Here's how the part is built. I have some questions about the finished solid (model axes, mm). A direction names the side the tool comes from. Coordinates: 2 decimals unless noted, no trailing zeros. Write each loop counter-clockwise with the first axis right and the second up, starting at its lowest first coordinate (ties: lowest second). Pieces come first, ordered by that corner, then holes. Notation, with made-up numbers: (82.25, 39.5) -> (122.25, 39.5) arc R22 cw to (122.25, 45.5) -> close; hole circle Ø9 at (8, -1.5). An arc over 180 degrees is marked (long way). Use a Markdown table: item, result. Add a question column.
Item 1: If I drill on line 1 along X through (y, z) = (3.6, 0); line 2 along Y through (x, z) = (20.75, 1.25); line 3 along Z through (x, y) = (13.25, 13), over which ranges is the centre line in solid material (lowest first)? Write a range as from..to.
Item 2: Imagine slicing it at A-A, the plane z = 0. Write out the boundary of the cut face in (x, y), and give its area (3 significant figures).
Item 3: On a 3-axis mill with a long thin cutter (end or side, diameter ignored), from which of +Z, -Z, +X, -X, +Y, -Y can I reach the whole of each face in a straight line? I mean faces 4 (the flat face through (11, 2, 5.715)), 5 (the cylindrical face through (14.415, 12.671, 1.58)). Say none if no direction works.
Item 4: Will these pins go through, and if not, where does the flat tip stop? pin 1 Ø1.5 at (x, z) = (1, -1.5) entering from +Y; pin 2 Ø8 at (x, y) = (10, 13) entering from +Z (3 decimals); pin 3 Ø1.5 at (x, z) = (0, 0) entering from -Y; pin 4 Ø5 at (y, z) = (5.5, 4) entering from +X.
Item 5: If we mould it in two halves opening along Y, with no side actions, what happens to faces 1 (the flat face through (10, 0, 0)), 2 (the cylindrical face through (12.11, 14.61, -4.7)), 3 (the cylindrical face through (-2.11, 2.25, 0.13))? For each: pulls with the +Y half, pulls with the -Y half, needs draft (parallel to the pull), parting line crosses it, or undercut.
Item 6: Imagine slicing it at C-C, the plane x = 0. Write out the boundary of the cut face in (y, z).
Item 7: Imagine slicing it at D-D, the plane z = -1.5. Write out the boundary of the cut face in (x, y).
```python
from build123d import *

# Parameters (mm, degrees)
SKETCH1_R               = 1.2192
BOSS_EXTRUDE1_DEPTH     = 4.572
SKETCH1_3_R             = 5.625
SKETCH1_3_R_2           = 4.125
BOSS_EXTRUDE2_DEPTH     = 21
SKETCH2_R               = 1.63195
CUT_EXTRUDE1_DEPTH      = 18.923
CUT_EXTRUDE1_DEPTH_BACK = 18.923


with BuildPart() as part:
    # Sketch1 → Boss-Extrude1 (new body)
    with BuildSketch(Plane(origin=(0, 0, 0), x_dir=(1, 0, 0), z_dir=(0, 1, 0))):
        with BuildLine():
            Line((3.6045, 5.715), (17.6045, 5.715))
            ThreePointArc((17.6045, 5.715), (23.3195, 0), (17.6045, -5.715))
            Line((17.6045, -5.715), (3.6045, -5.715))
            ThreePointArc((3.6045, -5.715), (-2.1105, 0), (3.6045, 5.715))
        make_face()
        Circle(SKETCH1_R, mode=Mode.SUBTRACT)
        with Locations((21.209, 0)):
            Circle(SKETCH1_R, mode=Mode.SUBTRACT)
    extrude(amount=BOSS_EXTRUDE1_DEPTH)

    # Sketch1_3 → Boss-Extrude2 (add)
    with BuildSketch(Plane(origin=(0, 0, 0), x_dir=(1, 0, 0), z_dir=(0, 1, 0))):
        with Locations((10.6045, 0)):
            Circle(SKETCH1_3_R)
        with Locations((10.6045, 0)):
            Circle(SKETCH1_3_R_2, mode=Mode.SUBTRACT)
    extrude(amount=BOSS_EXTRUDE2_DEPTH)

    # Sketch2 → Cut-Extrude1 (cut, two sides)
    with BuildSketch(Plane.XY) as cut_extrude1_sk:
        with Locations((10.6045, 15.24)):
            Circle(SKETCH2_R)
    extrude(amount=CUT_EXTRUDE1_DEPTH, mode=Mode.SUBTRACT)
    extrude(cut_extrude1_sk.sketch, amount=-CUT_EXTRUDE1_DEPTH_BACK, mode=Mode.SUBTRACT)


solid = part.part
```
Ans:
| question | item | result |
|---|---|---|
| 1 | line 1 | x = -2.11..-1.22, 1.22..19.99, 22.43..23.32 |
| 1 | line 2 | y = 0..4.57 |
| 1 | line 3 | z = -4.96..-3.16, 3.16..4.96 |
| 2 | outline | (-2.11, 0) -> (-1.22, 0) -> (-1.22, 4.57) -> (-2.11, 4.57) -> close; (1.22, 0) -> (19.99, 0) -> (19.99, 4.57) -> (16.23, 4.57) -> (16.23, 21) -> (14.73, 21) -> (14.73, 4.57) -> (6.48, 4.57) -> (6.48, 21) -> (4.98, 21) -> (4.98, 4.57) -> (1.22, 4.57) -> close; (22.43, 0) -> (23.32, 0) -> (23.32, 4.57) -> (22.43, 4.57) -> close |
| 2 | area | 143 mm^2 |
| 3 | face 4 | +Z, +X, -X, +Y, -Y |
| 3 | face 5 | +Y |
| 4 | pin 1 | stops at y = 4.57 |
| 4 | pin 2 | stops at z = 5.625 |
| 4 | pin 3 | passes through |
| 4 | pin 4 | stops at x = 23.07 |
| 5 | face 1 | pulls with the -Y half |
| 5 | face 2 | undercut |
| 5 | face 3 | needs draft |
| 6 | outline | (0, -4.43) -> (4.57, -4.43) -> (4.57, -1.22) -> (0, -1.22) -> close; (0, 1.22) -> (4.57, 1.22) -> (4.57, 4.43) -> (0, 4.43) -> close |
| 7 | outline | (-1.91, 0) -> (23.12, 0) -> (23.12, 4.57) -> (16.03, 4.57) -> (16.03, 21) -> (14.45, 21) -> (14.45, 4.57) -> (6.76, 4.57) -> (6.76, 21) -> (5.18, 21) -> (5.18, 4.57) -> (-1.91, 4.57) -> close |
